Verification items for this drawing (mm, ordinates from the low corner). A direction names the side the tool comes from. Coordinates: 2 decimals unless noted, no trailing zeros. Order: outer loops, then holes, each group sorted by start corner. A loop starts at its lowest first (then second) coordinate and runs counter-clockwise, first axis right, second up.
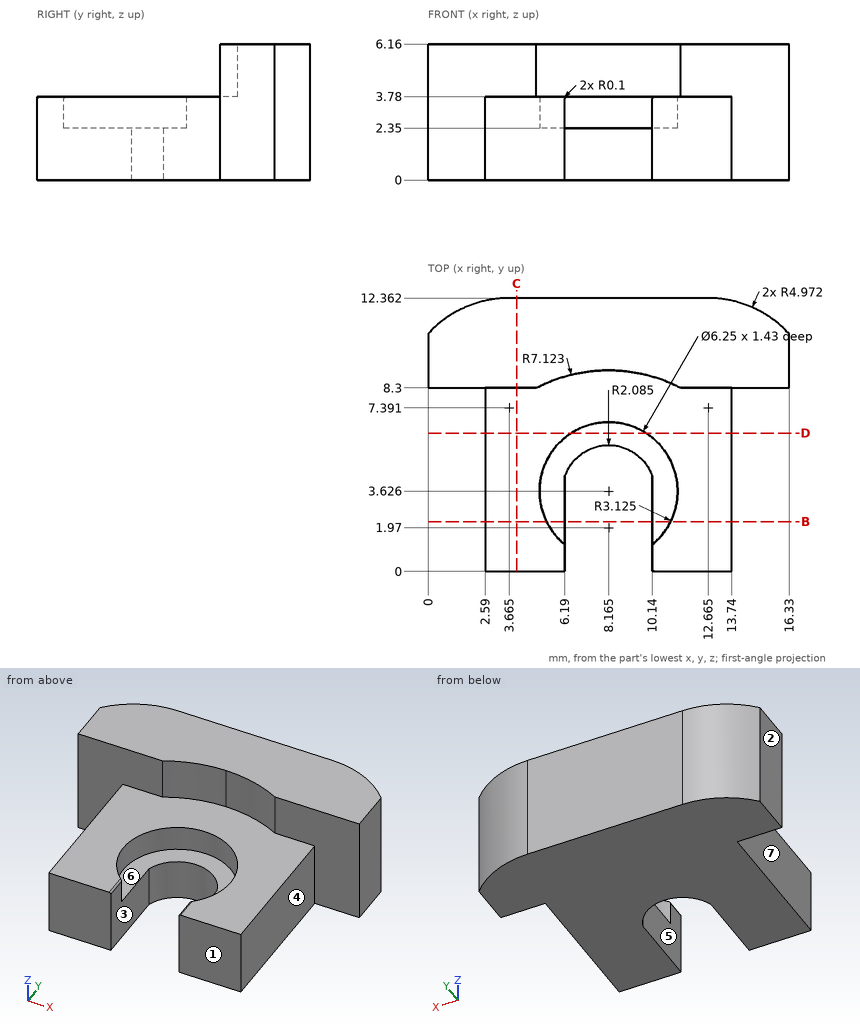
(1) Cross-section at D-D (y = 6.25). Enter the section's corners in (x, z), and give its area (3 significant figures).
Filled in:
outline: (2.59, 0) - (13.74, 0) - (13.74, 3.78) - (9.86, 3.78) - (9.86, 2.35) - (6.47, 2.35) - (6.47, 3.78) - (2.59, 3.78) - close
area: 37.3 mm2
(2) Release check for a two-part mould opening along X. For the marked faces 1, 2 and 3 record: +X half, -X half, draft (parallel to the pull), parting line (faces both ways), or undercut.
Filled in:
face 1: draft
face 2: -X half
face 3: undercut
(3) Tool access check on the marked faces 4, 5, 6 and 7. Record the directions out of +Z, -Z, +X, -X, +Y, -Y that give a thin tool (end or side, any length) a straight path to the whole face; none if there is none.
Filled in:
face 4: +Z, -Z, +X, -Y
face 5: +Z, -Z, -Y
face 6: +Z
face 7: +Z, -Z, -X, -Y
(4) Go/stop test with flat-tipped pins: P1, Ø4.5, axis at x = 11, y = 2.5, coming from the +Z side; P2, Ø3, axis at y = 6, z = 1.5, coming from the -X side; P3, Ø4.5, axis at x = 8.5, y = 3.5, coming from the +Z side. Record where each tip stops, or that it passes through.
Filled in:
P1: stops at z = 3.78
P2: stops at x = 2.59
P3: stops at z = 2.35
(5) Cross-section at C-C (x = 4). Enter the section's corners in (y, z), and give its area (3 significant figures).
Filled in:
outline: (0, 0) - (12.36, 0) - (12.36, 6.16) - (8.3, 6.16) - (8.3, 3.78) - (0, 3.78) - close
area: 56.4 mm2
(6) Thickness scan on probe 1 along X at (y, z) = (2, 1.5); probe 2 along Z at (x, y) = (5.5, 1); probe 3 along Y at (x, z) = (8.25, 4). Record the ranges inside material, lowest first.
Filled in:
probe 1: x = 2.59 to 6.19, 10.14 to 13.74
probe 2: z = 0 to 3.78
probe 3: y = 9.09 to 12.36
(7) Cross-section at B-B (y = 2.25). Enter the section's corners in (x, z).
Filled in:
outline: (2.59, 0) - (6.19, 0) - (6.19, 2.35) - (5.36, 2.35) - (5.36, 3.78) - (2.59, 3.78) - close; (10.14, 0) - (13.74, 0) - (13.74, 3.78) - (10.97, 3.78) - (10.97, 2.35) - (10.14, 2.35) - close
